```python
from build123d import *

# Parameters (mm, degrees)
EXTRUDE_1_DEPTH             = 198
CHAMFER_1_SIZE              = 11
HOLE_WIZARD_M41_AT_2_COUNT  = 2
HOLE_WIZARD_M41_AT_2_PITCH  = 35.0142828
HOLE_WIZARD_M41_AT_3_COUNT  = 2
HOLE_WIZARD_M41_AT_3_PITCH  = 75.00666637
HOLE_WIZARD_M42_AT_2_COUNT  = 2
HOLE_WIZARD_M42_AT_2_PITCH  = 103.004854255
HOLE_WIZARD_M42_AT_3_COUNT  = 2
HOLE_WIZARD_M42_AT_3_PITCH  = 143.003496461
HOLE_WIZARD_M51_D           = 5.8
HOLE_WIZARD_M51_DEPTH       = 3
HOLE_WIZARD_M51_CSINK_D     = 6
HOLE_WIZARD_M51_CSINK_ANGLE = 90
HOLE_WIZARD_M51_TIP         = 1.742495795
HOLE_WIZARD_M52_D           = 5.8
HOLE_WIZARD_M52_DEPTH       = 3
HOLE_WIZARD_M52_CSINK_D     = 6
HOLE_WIZARD_M52_CSINK_ANGLE = 90
HOLE_WIZARD_M52_TIP         = 1.742495795


with BuildPart() as part:
    # Эскиз1 → Бобышка-Вытянуть1 (new body)
    with BuildSketch(Plane.XY):
        Polygon((0, 0), (0, 15), (2, 15), (2, 2), (15, 2), (15, 0), align=None)
    extrude(amount=EXTRUDE_1_DEPTH)

    # Фаска1
    chamfer_1_edges = [part.edges().sort_by_distance(p)[0] for p in [
        (1, 15, 198),
        (1, 15, 0),
        (15, 1, 198),
        (15, 1, 0),
    ]]
    chamfer(chamfer_1_edges, length=CHAMFER_1_SIZE)

    # Эскиз2 → Зенковка для винта с потайной головкой M41 (revolve, cut)
    with BuildSketch(Plane(origin=(7, 0, 188), x_dir=(0, 0, -1), z_dir=(1, 0, 0))):
        Polygon((0, 0), (0, 2), (2.4, 2), (2.25, 1.85), (2.25, 1.45), (3.7, 0), align=None)
    hole_wizard_m41 = revolve(axis=Axis((7, -6.35, 188), (0, 1, 0)), mode=Mode.SUBTRACT)

    # Зенковка для винта с потайной головкой M41 at 2: Зенковка для винта с потайной головкой M41 ×2
    with Locations(*[Vector(0.028559774, 0, -0.999592086) * (i * HOLE_WIZARD_M41_AT_2_PITCH) for i in range(1, HOLE_WIZARD_M41_AT_2_COUNT)]):
        add(hole_wizard_m41, mode=Mode.SUBTRACT)

    # Зенковка для винта с потайной головкой M41 at 3: Зенковка для винта с потайной головкой M41 ×2
    with Locations(*[Vector(0.013332148, 0, -0.999911123) * (i * HOLE_WIZARD_M41_AT_3_PITCH) for i in range(1, HOLE_WIZARD_M41_AT_3_COUNT)]):
        add(hole_wizard_m41, mode=Mode.SUBTRACT)

    # Эскиз4 → Зенковка для винта с потайной головкой M42 (revolve, cut)
    with BuildSketch(Plane(origin=(0, 7, 10), x_dir=(0, 0, 1), z_dir=(0, 1, 0))):
        Polygon((0, 0), (0, 2), (2.4, 2), (2.25, 1.85), (2.25, 1.45), (3.7, 0), align=None)
    hole_wizard_m42 = revolve(axis=Axis((-6.35, 7, 10), (1, 0, 0)), mode=Mode.SUBTRACT)

    # Зенковка для винта с потайной головкой M42 at 2: Зенковка для винта с потайной головкой M42 ×2
    with Locations(*[Vector(0, 0.00970828, 0.999952874) * (i * HOLE_WIZARD_M42_AT_2_PITCH) for i in range(1, HOLE_WIZARD_M42_AT_2_COUNT)]):
        add(hole_wizard_m42, mode=Mode.SUBTRACT)

    # Зенковка для винта с потайной головкой M42 at 3: Зенковка для винта с потайной головкой M42 ×2
    with Locations(*[Vector(0, 0.006992836, 0.99997555) * (i * HOLE_WIZARD_M42_AT_3_PITCH) for i in range(1, HOLE_WIZARD_M42_AT_3_COUNT)]):
        add(hole_wizard_m42, mode=Mode.SUBTRACT)

    # Отверстие с зазором M51
    with Locations(Plane.ZY):
        with Locations((103, 8), (30, 8), (176, 8)):
            CounterSinkHole(HOLE_WIZARD_M51_D / 2, HOLE_WIZARD_M51_CSINK_D / 2, depth=HOLE_WIZARD_M51_DEPTH, counter_sink_angle=HOLE_WIZARD_M51_CSINK_ANGLE)
            with Locations((0, 0, -(HOLE_WIZARD_M51_DEPTH + HOLE_WIZARD_M51_TIP / 2))):  # 118° drill point
                Cone(0, HOLE_WIZARD_M51_D / 2, HOLE_WIZARD_M51_TIP, mode=Mode.SUBTRACT)

    # Отверстие с зазором M52
    with Locations(Plane.XZ):
        with Locations((8, 95), (8, 22), (8, 168)):
            CounterSinkHole(HOLE_WIZARD_M52_D / 2, HOLE_WIZARD_M52_CSINK_D / 2, depth=HOLE_WIZARD_M52_DEPTH, counter_sink_angle=HOLE_WIZARD_M52_CSINK_ANGLE)
            with Locations((0, 0, -(HOLE_WIZARD_M52_DEPTH + HOLE_WIZARD_M52_TIP / 2))):  # 118° drill point
                Cone(0, HOLE_WIZARD_M52_D / 2, HOLE_WIZARD_M52_TIP, mode=Mode.SUBTRACT)


solid = part.part
```
Model file for the job. Use its own axes, mm. Coordinates: 2 decimals unless noted, no trailing zeros. Order: outer loops, then holes, each group sorted by start corner. A loop starts at its lowest first (then second) coordinate and runs counter-clockwise, first axis right, second up. Notation, with made-up numbers: (28.5, 77) -> (66.5, 77) arc R4 cw to (66.5, 81) -> close; hole circle Ø5 at (85, -14.75). An arc over 180 degrees is marked (long way). Return JSON: item names as keys, results as strings.
Item 1: Wall check: line 1 along Y through (x, z) = (0.95, 176); line 2 along Y through (x, z) = (1.6, 113); line 3 along X through (y, z) = (3, 96.5). Give the ranges that are in metal, low to high. Write a range as from..to.
Model answer:
{"line 1": "y = 0..5.1, 10.9..15", "line 2": "y = 0..5.75, 10.25..15", "line 3": "x = 0..2"}
Item 2: Slice it at B-B (z = 41). Write the cut outline in (x, y).
Model answer:
{"outline": "(0, 0) -> (15, 0) -> (15, 2) -> (2, 2) -> (2, 15) -> (0, 15) -> close"}
Item 3: Slice it at A-A (z = 153). Write the cut outline in (x, y).
Model answer:
{"outline": "(0, 0) -> (4.3, 0) -> (5.75, 1.45) -> (5.75, 1.85) -> (5.6, 2) -> (2, 2) -> (2, 5.6) -> (1.85, 5.75) -> (1.45, 5.75) -> (0, 4.3) -> close; (0, 11.7) -> (1.45, 10.25) -> (1.85, 10.25) -> (2, 10.4) -> (2, 15) -> (0, 15) -> close; (10.25, 1.45) -> (11.7, 0) -> (15, 0) -> (15, 2) -> (10.4, 2) -> (10.25, 1.85) -> close"}
Item 4: Mould opens along Z. For faces 1 (the face through (1.06, 6.89, 27.32)), 2 (the face through (1.6, 1.6, 198)) say: pulls with the +Z half, pulls with the -Z half, needs draft (parallel to the pull), parting line crosses it, or undercut.
Model answer:
{"face 1": "undercut", "face 2": "pulls with the +Z half"}
Item 5: Pin check, flat tips, straight feed: P1, Ø6, axis at x = 8, z = 113, coming from the +Y side; P2, Ø3.5, axis at y = 8, z = 113, coming from the -X side; P3, Ø6.5, axis at y = 6.5, z = 71.5, coming from the +X side. Stop position of each tip, or through.
Model answer:
{"P1": "stops at y = 2", "P2": "passes through", "P3": "stops at x = 2"}
